Build history of the part. All positions in model axes, mm. A direction names the side the tool comes from. Coordinates: 2 decimals unless noted, no trailing zeros. Write each loop counter-clockwise with the first axis right and the second up, starting at its lowest first coordinate (ties: lowest second). Pieces come first, ordered by that corner, then holes.
from build123d import *

# Parameters (mm, degrees)
SKETCH3_W               = 20.828
SKETCH3_H               = 6.35
SKETCH3_W_2             = 4.572
SKETCH3_H_2             = 45.212
SKETCH3_W_3             = 150.876
BOSS_EXTRUDE1_DEPTH     = 38.1
SKETCH5_R               = 1.7272
SKETCH5_R_2             = 13
CUT_EXTRUDE2_DEPTH      = 193.753075911
CUT_EXTRUDE3_DEPTH      = 193.753075911
BOSS_EXTRUDE2_DEPTH     = 155.448
CUT_EXTRUDE1_DEPTH      = 120.492895555
CUT_EXTRUDE1_DEPTH_BACK = 120.492895555
SKETCH4_R               = 1.5875
SKETCH8_R               = 29.845
CUT_EXTRUDE4_DEPTH      = 193.75307593
BOSS_EXTRUDE3_DEPTH     = 20.828
SKETCH10_W              = 6.35
SKETCH10_H              = 38.1
CUT_EXTRUDE5_DEPTH      = 120.492895586


with BuildPart() as part:
    # Sketch3 → Boss-Extrude1 (new body)
    with BuildSketch(Plane(origin=(0, 0, 0), x_dir=(1, 0, 0), z_dir=(0, 1, 0))):
        with Locations((-90.424, -51.562)):
            Rectangle(SKETCH3_W, SKETCH3_H)
        with Locations((-77.724, -51.562)):
            Rectangle(SKETCH3_W_2, SKETCH3_H)
        with Locations((-77.724, -25.781)):
            Rectangle(SKETCH3_W_2, SKETCH3_H_2)
        with Locations((-77.724, 0)):
            Rectangle(SKETCH3_W_2, SKETCH3_H)
        Rectangle(SKETCH3_W_3, SKETCH3_H)
        with Locations((77.724, 0)):
            Rectangle(SKETCH3_W_2, SKETCH3_H)
        with Locations((77.724, -25.781)):
            Rectangle(SKETCH3_W_2, SKETCH3_H_2)
        with Locations((77.724, -51.562)):
            Rectangle(SKETCH3_W_2, SKETCH3_H)
        with Locations((90.424, -51.562)):
            Rectangle(SKETCH3_W, SKETCH3_H)
    extrude(amount=BOSS_EXTRUDE1_DEPTH)

    # Sketch5 → Cut-Extrude2 (cut, through all)
    with BuildSketch(Plane.ZY.offset(80.01)):
        with Locations((9.225, 32.05)):
            Circle(SKETCH5_R)
        with Locations((35.225, 32.05)):
            Circle(SKETCH5_R)
        with Locations((35.225, 6.05)):
            Circle(SKETCH5_R)
        with Locations((9.225, 6.05)):
            Circle(SKETCH5_R)
        with Locations((22.225, 19.05)):
            Circle(SKETCH5_R_2)
    extrude(amount=-CUT_EXTRUDE2_DEPTH, mode=Mode.SUBTRACT)

    # Sketch6 → Cut-Extrude3 (cut, through all)
    with BuildSketch(Plane.ZY.offset(80.01)):
        with BuildLine():
            Line((22.225, 45.72), (-24.944215418, 45.72))
            Line((-24.944215418, 45.72), (-24.944215418, -7.62))
            Line((-24.944215418, -7.62), (22.225, -7.62))
            ThreePointArc((22.225, -7.62), (-4.445, 19.05), (22.225, 45.72))
        make_face()
    extrude(amount=-CUT_EXTRUDE3_DEPTH, mode=Mode.SUBTRACT)

    # Sketch7 → Boss-Extrude2 (add)
    with BuildSketch(Plane.ZY.offset(80.01)):
        with BuildLine():
            Line((3.55988816, 38.1), (10.7773747, 38.1))
            ThreePointArc((10.7773747, 38.1), (0, 19.05), (10.7773747, 0))
            Line((10.7773747, 0), (3.55988816, 0))
            ThreePointArc((3.55988816, 0), (-0.473774796, 5.048052894), (-3.175, 10.918032218))
            Line((-3.175, 10.918032218), (-3.175, 27.181967782))
            ThreePointArc((-3.175, 27.181967782), (-0.473774796, 33.051947106), (3.55988816, 38.1))
        make_face()
    extrude(amount=-BOSS_EXTRUDE2_DEPTH)

    # Sketch4 → Cut-Extrude1 (cut, two sides: drawn at the far end of the back side and taken through both)
    with BuildSketch(Plane.XY.offset(3.175).offset(-CUT_EXTRUDE1_DEPTH_BACK)):
        Polygon((17.399, 25.4), (17.399, 19.05), (17.399, 12.7), (23.749, 12.7), (23.749, 25.4), align=None)
        Polygon((-17.399, 25.4), (-23.749, 25.4), (-23.749, 12.7), (-17.399, 12.7), (-17.399, 19.05), align=None)
        with Locations((-20.574, 31.75)):
            Circle(SKETCH4_R)
        with Locations((-20.574, 6.35)):
            Circle(SKETCH4_R)
        with Locations((20.574, 6.35)):
            Circle(SKETCH4_R)
        with Locations((20.574, 31.75)):
            Circle(SKETCH4_R)
    extrude(amount=CUT_EXTRUDE1_DEPTH + CUT_EXTRUDE1_DEPTH_BACK, mode=Mode.SUBTRACT)

    # Sketch8 → Cut-Extrude4 (cut, through all)
    with BuildSketch(Plane.ZY.offset(80.01)):
        with Locations((22.225, 19.05)):
            Circle(SKETCH8_R)
    cut_extrude4 = extrude(amount=CUT_EXTRUDE4_DEPTH, mode=Mode.SUBTRACT)

    # Sketch9 → Boss-Extrude3 (add)
    with BuildSketch(Plane.ZY.offset(80.01)):
        with BuildLine():
            Line((48.387, 38.1), (48.387, 33.412234541))
            ThreePointArc((48.387, 33.412234541), (46.904737017, 35.831972642), (45.199366694, 38.1))
            Line((45.199366694, 38.1), (48.387, 38.1))
        make_face()
        with BuildLine():
            Line((48.387, 0), (48.387, 4.687765459))
            ThreePointArc((48.387, 4.687765459), (46.904737017, 2.268027358), (45.199366694, 0))
            Line((45.199366694, 0), (48.387, 0))
        make_face()
    boss_extrude3 = extrude(amount=BOSS_EXTRUDE3_DEPTH)

    # Mirror4: Cut-Extrude4, Boss-Extrude3 across plane
    add(cut_extrude4.mirror(Plane(origin=(0, 0, 0), x_dir=(0, 0, 1), z_dir=(1, 0, 0))), mode=Mode.SUBTRACT)
    add(boss_extrude3.mirror(Plane(origin=(0, 0, 0), x_dir=(0, 0, 1), z_dir=(1, 0, 0))))

    # Sketch10 → Cut-Extrude5 (cut, through all)
    with BuildSketch(Plane.XY.offset(3.175)):
        with Locations((-20.574, 19.05)):
            Rectangle(SKETCH10_W, SKETCH10_H)
        with Locations((20.574, 19.05)):
            Rectangle(SKETCH10_W, SKETCH10_H)
    extrude(amount=CUT_EXTRUDE5_DEPTH, mode=Mode.SUBTRACT)


solid = part.part
(1) Slice it at A-A, the plane z = 40. List the corners of the cut face in (x, y), and give its area (3 significant figures).
(2) Slice it at D-D, the plane z = 16.5. List the corners of the cut face in (x, y).
(3) Probe L1, parallel to X at y = 18, z = 2; L2, parallel to X at y = 4, z = 52; L3, parallel to Z at x = -78, y = 6. List the from-to ranges inside material, lowest first.
(4) Slice it at B-B, the plane y = 16.5. List the corners of the cut face in (x, z) (3 decimals), and give its area (3 significant figures).
(5) Two-plate mould, pull along Z, no slides. Class faces 1 (the flat face through (1, 19, -3.175)), 2 (the cylindrical face through (-77.76, 6.57, 36.87)), 3 (the flat face through (-23.749, 36, 5)): pulls with the +Z half, pulls with the -Z half, needs draft (parallel to the pull), parting line crosses it, or undercut.
(6) 3-axis set-ups, long thin cutter, end or side, ignore diameter. For faces 4 (the cylindrical face through (-1.12, 4.971, -0.426)), 5 (the flat face through (-100.838, 19, 53)), 6 (the cylindrical face through (-0.244, 34.819, 6.563)), 7 (the flat face through (-17.399, 36, 5)), 8 (the flat face through (21, 12.7, 0)): which of +Z, -Z, +X, -X, +Y, -Y reach the whole face in a straight line?
(7) Slice it at C-C, the plane x = 60. List the corners of the cut face in (y, z) (3 decimals), and give its area (3 significant figures).
(8) Flat gauge pins, fed straight in: P1, Ø3, axis at y = 19.5, z = 37, coming from the +X side; P2, Ø6, axis at y = 34, z = 7, coming from the -X side; P3, Ø1.9, axis at x = 20.574, y = 6.35, coming from the +Z side; P4, Ø1.9, axis at x = -20.5, z = 0.5, coming from the -Y side. Where does each tip first touch, or does it go through?
Results:
1. outline: (-80.01, 0) - (-75.44, 0) - (-75.44, 38.1) - (-80.01, 38.1) - close; (75.44, 0) - (80.01, 0) - (80.01, 38.1) - (75.44, 38.1) - close
1. area: 348 mm2
2. outline: (-80.01, 0) - (-75.44, 0) - (-75.44, 7.38) - (-80.01, 7.38) - close; (-80.01, 30.72) - (-75.44, 30.72) - (-75.44, 38.1) - (-80.01, 38.1) - close; (75.44, 0) - (80.01, 0) - (80.01, 7.38) - (75.44, 7.38) - close; (75.44, 30.72) - (80.01, 30.72) - (80.01, 38.1) - (75.44, 38.1) - close
3. L1: x = -80.01 to -23.75, -17.4 to 17.4, 23.75 to 80.01
3. L2: x = -100.84 to -75.44, 75.44 to 100.84
3. L3: z = -1.03 to 7.5, 10.95 to 33.5, 36.95 to 54.74
4. outline: (-100.838, 51.961) - (-80.01, 51.961) - (-80.01, 34.972) - (-75.438, 34.972) - (-75.438, 54.737) - (-100.838, 54.737) - close; (-80.01, -3.175) - (-23.749, -3.175) - (-23.749, 3.175) - (-75.438, 3.175) - (-75.438, 9.478) - (-80.01, 9.478) - close; (-17.399, -3.175) - (17.399, -3.175) - (17.399, 3.175) - (-17.399, 3.175) - close; (23.749, -3.175) - (80.01, -3.175) - (80.01, 9.478) - (75.438, 9.478) - (75.438, 3.175) - (23.749, 3.175) - close; (75.438, 34.972) - (80.01, 34.972) - (80.01, 51.961) - (100.838, 51.961) - (100.838, 54.737) - (75.438, 54.737) - close
4. area: 1,290 mm2
5. face 1: pulls with the -Z half
5. face 2: undercut
5. face 3: needs draft
6. face 4: -Z, +X, -X, -Y
6. face 5: +Z, -Z, -X, +Y, -Y
6. face 6: +Z
6. face 7: +Z, +Y, -Y
6. face 8: +Z, -Z
7. outline: (0, 3.56) arc R26.67 ccw to (10.918, -3.175) - (27.182, -3.175) arc R26.67 ccw to (38.1, 3.56) - (38.1, 10.777) arc R22.225 cw to (30.498, 3.175) - (7.602, 3.175) arc R22.225 cw to (0, 10.777) - close
7. area: 230 mm2
8. P1: stops at x = 80.01
8. P2: stops at x = -80.01
8. P3: passes through
8. P4: stops at y = 2.33
